Study the drawing (mm; zero at the part's minimum x, y, z) and answer. Coordinates: 2 decimals unless noted, no trailing zeros. Loops run counter-clockwise (first coordinate to the right, second up) from the corner with the lowest first, then second, coordinate; pieces in that order, holes last. Notation, with made-up numbers: (17.5, -5) - (49.5, -5) arc R19 cw to (49.5, 12) - close; hole circle Ø4 at (-21, -11.5). An arc over 180 degrees is marked (long way). Write each question's results on one line, items separated by ' | '. Start each with the question number.
(1) Find section A-A on y = 5. Determine the outline of the cut face in (x, z), then the cut area to 3 significant figures.
(2) Given pin 1 Ø1.5 at (x, y) = (2.5, 23) entering from -Z, flat-ended and moving along its own axis, determine where the tip first touches the part or whether it passes through.
(3) Consider line 1 (Y direction, x = 2.6, z = 5); line 2 (X direction, y = 37, z = 8.5); line 3 (Z direction, x = 3.4, y = 5). Determine where each line is inside the solid, lowest interval first. Write a range as from..to.
(4) Find section C-C on z = 1. Determine the outline of the cut face in (x, y).
(5) Determine the mould class of the marked faces 1, 2, 3 and 4 for opening direction Z: released by +Z, released by -Z, zero draft, split by the parting line, or undercut.
(6) Find section D-D on x = 0.4. Determine the outline of the cut face in (y, z), then the cut area to 3 significant figures.
(7) Find section B-B on x = 3.05. Determine the outline of the cut face in (y, z), then the cut area to 3 significant figures.
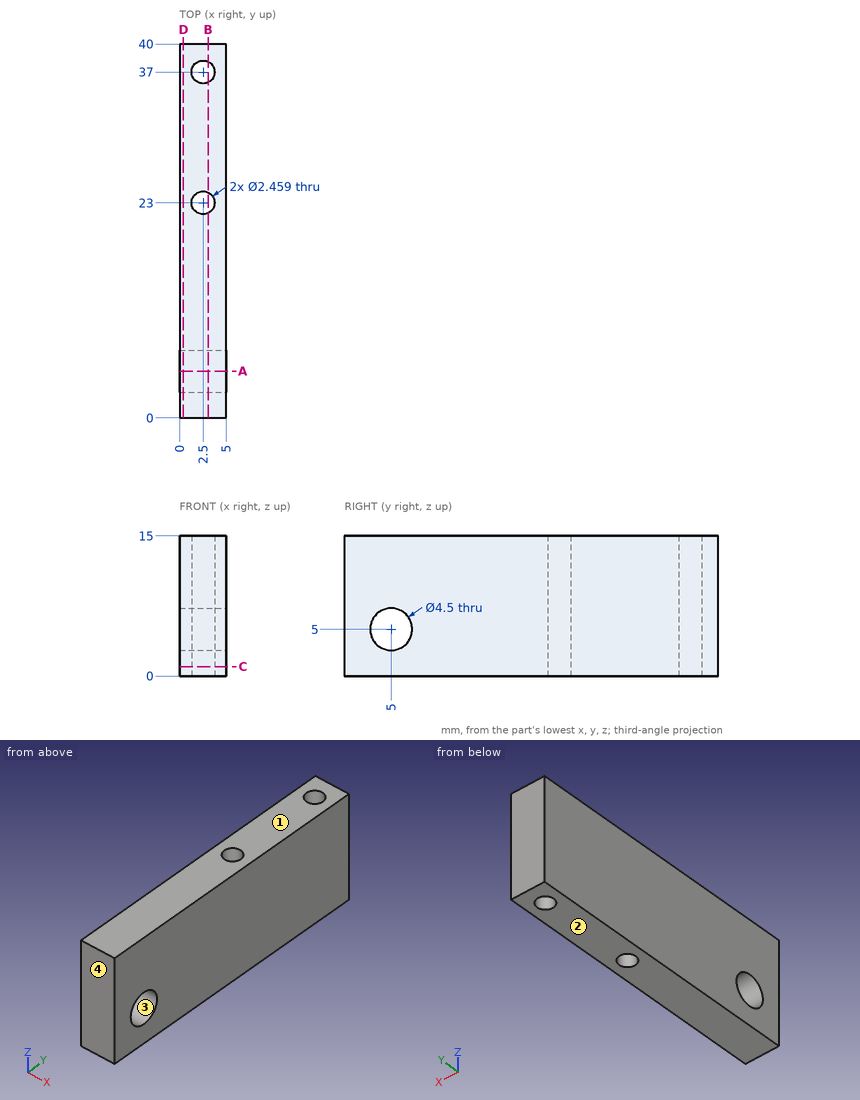
Values:
1) outline: (0, 0) - (5, 0) - (5, 2.75) - (0, 2.75) - close; (0, 7.25) - (5, 7.25) - (5, 15) - (0, 15) - close | area: 52.5 mm²
2) pin 1: passes through
3) line 1: y = 0..2.75, 7.25..21.77, 24.23..35.77, 38.23..40 | line 2: x = 0..1.27, 3.73..5 | line 3: z = 0..2.75, 7.25..15
4) outline: (0, 0) - (5, 0) - (5, 40) - (0, 40) - close; hole circle Ø2.46 at (2.5, 23); hole circle Ø2.46 at (2.5, 37)
5) face 1: released by +Z | face 2: released by -Z | face 3: undercut | face 4: zero draft
6) outline: (0, 0) - (40, 0) - (40, 15) - (0, 15) - close; hole circle Ø4.5 at (5, 5) | area: 584 mm²
7) outline: (0, 0) - (21.9, 0) - (21.9, 15) - (0, 15) - close; (24.1, 0) - (35.9, 0) - (35.9, 15) - (24.1, 15) - close; (38.1, 0) - (40, 0) - (40, 15) - (38.1, 15) - close; hole circle Ø4.5 at (5, 5) | area: 518 mm²
